Geometry: final body of the model. Coordinates: model frame, mm. A direction names the side the tool comes from. Give positions to 0.01 mm unless a question says otherwise; leave off trailing zeros. Order: outer loops, then holes, each group sorted by start corner. A loop starts at its lowest first (then second) coordinate and runs counter-clockwise, first axis right, second up. Notation, with made-up numbers: (77, -3) -> (106, -3) arc R24 ccw to (106, 13) -> close; hole circle Ø10 at (21.25, -4.5). An arc over 180 degrees is marked (long way). One line per question, with ' | ' between items. Start each with the question number.
(1) Ray query, L1, parallel to Y at x = 0, z = -2.4; L2, parallel to Y at x = 0, z = 1.25. Return the intervals inside material, ascending.
(2) Section C-C (x = 3). Return loops of the section in (y, z).
(3) First-contact query: pin 1 Ø1 at (x, y) = (2, -2.5) entering from -Z; pin 2 Ø1 at (y, z) = (2, 0) entering from +X; pin 3 Ø3 at (x, z) = (3.5, -0.5) entering from -Y. Flat tips, straight axial feed; report the tip coordinate or a pass-through.
(4) Section A-A (y = 0). Return loops of the section in (x, z), then the cut area to 3 significant figures.
(5) Set-up query: faces 3 (the face through (1, -2, -2.2)), 4 (the face through (0.07, -1.5, -0.04)). Return all of +Z, -Z, +X, -X, +Y, -Y with unobstructed straight access to the full face (end or side cutting, diameter ignored); none if empty.
(6) Mould query, pull axis Y, two halves, no side actions, for faces 1 (the face through (4.88, -1.08, 0.04)), 2 (the face through (1, 2, 2.2)). Classes: +Y half, -Y half, draft (parallel to the pull), parting line (faces both ways), or undercut.
Autodesk Inventor part; units mm, degrees
ref_plane "YZ Plane" through (0, 0, 0) normal (1, 0, 0) x (0, 1, 0)
ref_plane "XZ Plane" through (0, 0, 0) normal (0, 1, 0) x (-1, 0, 0)
ref_plane "XY Plane" through (0, 0, 0) normal (0, 0, 1) x (1, 0, 0)
sketch "Sketch1" plane through (0, 0, 0) normal (1, 0, 0) x (0, 1, 0)
  line L0 (5, 0) -> (1.5, 0)
  line L1 (1.5, 0) -> (1.5, -2.5)
  line L2 (5, -2.5) -> (5, 0)
  line L3 (-1, 0) -> (6, 0)
  line L4 (0, -3) -> (0, 0.5)
  line L5 (1.5, -2.5) -> (2, -2.5)
  line L6 (2, -2.5) -> (2, -2.2)
  line L7 (2, -2.2) -> (4, -2.2)
  line L8 (4, -2.2) -> (4, -2.5)
  line L9 (4, -2.5) -> (5, -2.5)
  point P0 (0, 0)
  point P1 (4, -2.35)
  point P2 (2, -2.35)
  dimension "d1" = 5
  dimension "d2" = 1.5
  dimension "d5" = 2.2
  dimension "d6" = 1
  dimension "d7" = 0.5
  dimension "d9" = 2.5
revolve "Revolution1" add sketch "Sketch1" angle 360 about axis through (0, 0, -10) along (0, 0, 1)
mirror "Mirror1" about plane through (0, 0, 0) normal (0, 0, 1) of "Revolution1"
properties part number "Bearing_BS69310-5"
Response:
1) L1: y = -5 to -4, -2 to -1.5, 1.5 to 2, 4 to 5 | L2: y = -5 to -1.5, 1.5 to 5
2) outline: (-4, -2.5) -> (-2.65, -2.5) -> (-2.65, -2.2) -> (2.65, -2.2) -> (2.65, -2.5) -> (4, -2.5) -> (4, 2.5) -> (2.65, 2.5) -> (2.65, 2.2) -> (-2.65, 2.2) -> (-2.65, 2.5) -> (-4, 2.5) -> close
3) pin 1: stops at z = -2.2 | pin 2: stops at x = 4.77 | pin 3: stops at y = -4.58
4) outline: (-5, -2.5) -> (-4, -2.5) -> (-4, -2.2) -> (-2, -2.2) -> (-2, -2.5) -> (-1.5, -2.5) -> (-1.5, 2.5) -> (-2, 2.5) -> (-2, 2.2) -> (-4, 2.2) -> (-4, 2.5) -> (-5, 2.5) -> close; (1.5, -2.5) -> (2, -2.5) -> (2, -2.2) -> (4, -2.2) -> (4, -2.5) -> (5, -2.5) -> (5, 2.5) -> (4, 2.5) -> (4, 2.2) -> (2, 2.2) -> (2, 2.5) -> (1.5, 2.5) -> close | area: 32.6 mm^2
5) face 3: -Z | face 4: +Z, -Z
6) face 1: parting line | face 2: undercut
